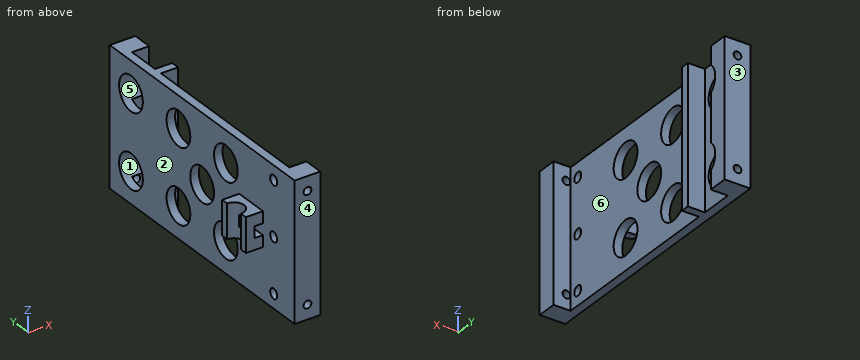
```python
from build123d import *

# Parameters (mm, degrees)
F0_W      = 9
F0_H      = 93.5
F1_DEPTH  = 48
F2_R      = 1.35
F3_DEPTH  = 8
F4_R      = 1.35
F5_DEPTH  = 8
F6_R      = 1.75
F7_DEPTH  = 9.001
F8_R      = 6
F9_DEPTH  = 9.001
F10_W     = 6
F10_H     = 64.9
F10_H_2   = 11.6
F11_DEPTH = 48.001
F12_W     = 12
F12_H     = 12
F13_DEPTH = 6
F14_W     = 3
F14_H     = 4
F15_DEPTH = 12
F16_R     = 3.5
F17_DEPTH = 30.001


with BuildPart() as f1:
    # F0 (on Top) → F1 (new body)
    with BuildSketch(Plane.XY):
        Rectangle(F0_W, F0_H)
    extrude(amount=F1_DEPTH)

    # F2 (on face) → F3 (cut)
    with BuildSketch(Plane.XZ.offset(46.75)):
        with Locations((0, 43)):
            Circle(F2_R)
        with Locations((0, 5)):
            Circle(F2_R)
    extrude(amount=-F3_DEPTH, mode=Mode.SUBTRACT)

    # F4 (on face) → F5 (cut)
    with BuildSketch(Plane(origin=(0, 46.75, 0), x_dir=(-1, 0, 0), z_dir=(0, 1, 0))):
        with Locations((0, 43)):
            Circle(F4_R)
        with Locations((0, 5)):
            Circle(F4_R)
    extrude(amount=-F5_DEPTH, mode=Mode.SUBTRACT)

    # F6 (on face) → F7 (cut, through all)
    with BuildSketch(Plane.YZ.offset(4.5)):
        with Locations((-36.15, 43)):
            Circle(F6_R)
        with Locations((-36.15, 24)):
            Circle(F6_R)
        with Locations((-36.15, 5)):
            Circle(F6_R)
    extrude(amount=-F7_DEPTH, mode=Mode.SUBTRACT)

    # F8 (on face) → F9 (cut, through all)
    with BuildSketch(Plane.YZ.offset(4.5)):
        with Locations((-12, 11)):
            Circle(F8_R)
        with Locations((0, 24)):
            Circle(F8_R)
        with Locations((-12, 37)):
            Circle(F8_R)
        with Locations((12, 11)):
            Circle(F8_R)
        with Locations((12, 37)):
            Circle(F8_R)
        with Locations((36, 11)):
            Circle(F8_R)
        with Locations((36, 37)):
            Circle(F8_R)
    extrude(amount=-F9_DEPTH, mode=Mode.SUBTRACT)

    # F10 (on face) → F11 (cut, through all)
    with BuildSketch(Plane.XY.offset(48)):
        with Locations((1.5, -7.3)):
            Rectangle(F10_W, F10_H)
        with Locations((1.5, 33.95)):
            Rectangle(F10_W, F10_H_2)
    extrude(amount=-F11_DEPTH, mode=Mode.SUBTRACT)

    # F12 (on face) → F13 (join)
    with BuildSketch(Plane(origin=(-4.5, 0, 0), x_dir=(0, -1, 0), z_dir=(-1, 0, 0))):
        with Locations((24.75, 24)):
            Rectangle(F12_W, F12_H)
    extrude(amount=F13_DEPTH)

    # F14 (on face) → F15 (cut, through all)
    with BuildSketch(Plane.XZ.offset(30.75)):
        with Locations((-6, 23.958516)):
            Rectangle(F14_W, F14_H)
    extrude(amount=-F15_DEPTH, mode=Mode.SUBTRACT)

    # F16 (on face) → F17 (cut, through all)
    with BuildSketch(Plane.XY.offset(30)):
        with Locations((-10.5, -24.75)):
            Circle(F16_R)
    extrude(amount=-F17_DEPTH, mode=Mode.SUBTRACT)


solid = f1.part
```
Part model, mm, in its own coordinate system. Face numbers are marked on the shaded views. A direction names the side the tool comes from. Round coordinates to 2 decimals unless told otherwise and drop trailing zeros. Write each loop counter-clockwise with the first axis right and the second up, starting at its lowest first coordinate (ties: lowest second). Pieces come first, ordered by that corner, then holes. Notation, with made-up numbers: M -10.5,13.5 L 16.5,13.5 A16 cw 16.5,28.5 Z; hole C 45,6.5 d5. An arc over 180 degrees is marked long. Answer as CSV lines item,"result". Start each with the question number.
1) Drop flat-ended pins along their axis: pin 1 (2 mm diameter, centred on y = -21, z = 24, fed in from +X); pin 2 (1 mm diameter, centred on x = 0, y = 31, fed in from -Z); pin 3 (15.5 mm diameter, centred on y = 36, z = 11, fed in from -X); pin 4 (5 mm diameter, centred on x = -9, z = 25.5, fed in from -Y). Give the stop position or say it passes through.
2) Band-saw the part on A-A (y = 12). List the corners of the cut face in (x, z), then the cut area to 3 significant figures.
3) Band-saw the part on B-B (z = 11). List the corners of the cut face in (x, y).
4) Mould opens along Y. For the marked faces 1, 2, 3 and 4 say: +Y half, -Y half, draft (parallel to the pull), parting line (faces both ways), or undercut.
5) Band-saw the part on D-D (x = 3.25). List the corners of the cut face in (y, z), then the cut area to 3 significant figures.
6) Which spindle directions (+Z, -Z, +X, -X, +Y, -Y) get a long thin tool onto all of the face, cutting with end or side? Do the marked faces 5 and 6. Say none if no direction does.
7) Drill centre lines: L1, parallel to Z at x = -2.45, y = 12; L2, parallel to Z at x = 0, y = -44.75; L3, parallel to Y at x = 0, z = 19.5. Where is each one in solid material? Low to high.
8) Band-saw the part on C-C (x = -3.25). Count the separate pieces of the cut face and the enclosed holes in it, then the cut area to 3 significant figures.
Worked out:
1,pin 1,"x = -1.5"
1,pin 2,"through"
1,pin 3,"x = -4.5"
1,pin 4,"y = -30.75"
2,outline,"M -4.5,0 L -1.5,0 L -1.5,5 L -4.5,5 Z; M -4.5,17 L -1.5,17 L -1.5,31 L -4.5,31 Z; M -4.5,43 L -1.5,43 L -1.5,48 L -4.5,48 Z"
2,area,"72.0 mm²"
3,outline,"M -4.5,-46.75 L 4.5,-46.75 L 4.5,-39.75 L -1.5,-39.75 L -1.5,-18 L -4.5,-18 Z; M -4.5,-6 L -1.5,-6 L -1.5,6 L -4.5,6 Z; M -4.5,18 L -1.5,18 L -1.5,25.15 L 4.5,25.15 L 4.5,28.15 L -1.5,28.15 L -1.5,30 L -4.5,30 Z; M -4.5,42 L 4.5,42 L 4.5,46.75 L -4.5,46.75 Z"
4,face 1,"undercut"
4,face 2,"draft"
4,face 3,"+Y half"
4,face 4,"-Y half"
5,outline,"M -46.75,0 L -39.75,0 L -39.75,48 L -46.75,48 Z; M 25.15,0 L 28.15,0 L 28.15,48 L 25.15,48 Z; M 39.75,0 L 46.75,0 L 46.75,48 L 39.75,48 L 39.75,41.68 A6 cw 39.75,32.32 L 39.75,15.68 A6 cw 39.75,6.32 Z"
5,area,"787 mm²"
6,face 5,"+X, -X"
6,face 6,"+Z, -Z, +X"
7,L1,"0 to 5, 17 to 31, 43 to 48"
7,L2,"0 to 3.65, 6.35 to 41.65, 44.35 to 48"
7,L3,"-46.75 to -39.75, 25.15 to 28.15, 39.75 to 46.75"
8,separate pieces,"1"
8,enclosed holes,"10"
8,area,"3,670 mm²"
